```python
from build123d import *

# Parameters (mm, degrees)
SKETCH1_W                   = 60
SKETCH1_H                   = 60
BOSS_EXTRUDE1_DEPTH         = 45
BOSS_EXTRUDE2_DEPTH         = 34
SKETCH3_R                   = 3.5
BOSS_EXTRUDE3_DEPTH         = 4
SKETCH4_R                   = 4.5
BOSS_EXTRUDE4_DEPTH         = 1.5
SKETCH5_R                   = 0.5
BOSS_EXTRUDE5_DEPTH         = 8.5
SKETCH6_R                   = 27
CUT_EXTRUDE1_DEPTH          = 0.3
SKETCH7_R                   = 12
BOSS_EXTRUDE6_DEPTH         = 3.3
SKETCH8_R                   = 4
BOSS_EXTRUDE7_DEPTH         = 29
CUT_EXTRUDE2_DEPTH          = 109.592080743
CUT_EXTRUDE2_DEPTH_BACK     = 109.592080743
M4_TAPPED_HOLE1_D           = 3.3
M4_TAPPED_HOLE1_DEPTH       = 10.1
M4_TAPPED_HOLE1_CSINK_D     = 4
M4_TAPPED_HOLE1_CSINK_ANGLE = 90
M4_TAPPED_HOLE1_TIP         = 0.991420021
FILLET1_R                   = 3.5
FILLET2_R                   = 4
FILLET3_R                   = 5.7


with BuildPart() as part:
    # Sketch1 → Boss-Extrude1 (new body)
    with BuildSketch(Plane(origin=(0, 0, 0), x_dir=(0, 0, -1), z_dir=(1, 0, 0))):
        with Locations((30, 0)):
            Rectangle(SKETCH1_W, SKETCH1_H)
    extrude(amount=-BOSS_EXTRUDE1_DEPTH)

    # Sketch2 → Boss-Extrude2 (add)
    with BuildSketch(Plane.ZY.offset(45)):
        Polygon((-1.8, 16.87), (-1.8, -16.87), (-10.698224855, -19.301775145), (-13.13, -28.2), (-46.87, -28.2), (-49.301775145, -19.301775145), (-58.2, -16.87), (-58.2, 16.87), (-49.301775145, 19.301775145), (-46.87, 28.2), (-13.13, 28.2), (-10.698224855, 19.301775145), align=None)
    extrude(amount=BOSS_EXTRUDE2_DEPTH)

    # Sketch3 → Boss-Extrude3 (add)
    with BuildSketch(Plane.ZY.offset(45)):
        with Locations((-5.251262658, 24.748737342)):
            Circle(SKETCH3_R)
        with Locations((-5.251262658, -24.748737342)):
            Circle(SKETCH3_R)
        with Locations((-54.748737342, -24.748737342)):
            Circle(SKETCH3_R)
        with Locations((-54.748737342, 24.748737342)):
            Circle(SKETCH3_R)
    extrude(amount=BOSS_EXTRUDE3_DEPTH)

    # Sketch4 → Boss-Extrude4 (add)
    with BuildSketch(Plane(origin=(0, 0, -58.2), x_dir=(-1, 0, 0), z_dir=(0, 0, -1))):
        with Locations(Location((71, 0, 0), (0, 0, 180))):
            Circle(SKETCH4_R)
    extrude(amount=BOSS_EXTRUDE4_DEPTH)

    # Sketch5 → Boss-Extrude5 (add)
    with BuildSketch(Plane(origin=(0, 0, -59.7), x_dir=(-1, 0, 0), z_dir=(0, 0, -1))):
        with Locations((73, -2)):
            Circle(SKETCH5_R)
        with Locations((73, 0)):
            Circle(SKETCH5_R)
        with Locations((73, 2)):
            Circle(SKETCH5_R)
        with Locations((69, -2)):
            Circle(SKETCH5_R)
        with Locations((69, 0)):
            Circle(SKETCH5_R)
        with Locations((69, 2)):
            Circle(SKETCH5_R)
    extrude(amount=BOSS_EXTRUDE5_DEPTH)

    # Sketch6 → Cut-Extrude1 (cut)
    with BuildSketch(Plane(origin=(0, 0, 0), x_dir=(0, 0, -1), z_dir=(1, 0, 0))):
        with Locations((30, 0)):
            Circle(SKETCH6_R)
    extrude(amount=-CUT_EXTRUDE1_DEPTH, mode=Mode.SUBTRACT)

    # Sketch7 → Boss-Extrude6 (add)
    with BuildSketch(Plane(origin=(-0.3, 0, 0), x_dir=(0, 0, -1), z_dir=(1, 0, 0))):
        with Locations((20, 0)):
            Circle(SKETCH7_R)
    extrude(amount=BOSS_EXTRUDE6_DEPTH)

    # Sketch8 → Boss-Extrude7 (add)
    with BuildSketch(Plane(origin=(3, 0, 0), x_dir=(0, 0, -1), z_dir=(1, 0, 0))):
        with Locations(Location((20, 0, 0), (0, 0, 180))):
            Circle(SKETCH8_R)
    extrude(amount=BOSS_EXTRUDE7_DEPTH)

    # Sketch9 → Cut-Extrude2 (cut, two sides: drawn at the far end of the back side and taken through both)
    with BuildSketch(Plane(origin=(0, 0, 0), x_dir=(1, 0, 0), z_dir=(0, 1, 0)).offset(-CUT_EXTRUDE2_DEPTH_BACK)):
        with BuildLine():
            Line((32, 17), (20, 17))
            ThreePointArc((20, 17), (17.4, 16.747644855), (14.897059671, 16))
            Line((14.897059671, 16), (32, 16))
            Line((32, 16), (32, 17))
        make_face()
    extrude(amount=CUT_EXTRUDE2_DEPTH + CUT_EXTRUDE2_DEPTH_BACK, mode=Mode.SUBTRACT)

    # M4 Tapped Hole1
    with Locations(Plane(origin=(0, 0, 0), x_dir=(0, 0, -1), z_dir=(1, 0, 0))):
        with Locations((5.251262658, -24.748737342), (5.251262658, 24.748737342), (54.748737342, -24.748737342), (54.748737342, 24.748737342)):
            CounterSinkHole(M4_TAPPED_HOLE1_D / 2, M4_TAPPED_HOLE1_CSINK_D / 2, depth=M4_TAPPED_HOLE1_DEPTH, counter_sink_angle=M4_TAPPED_HOLE1_CSINK_ANGLE)
            with Locations((0, 0, -(M4_TAPPED_HOLE1_DEPTH + M4_TAPPED_HOLE1_TIP / 2))):  # 118° drill point
                Cone(0, M4_TAPPED_HOLE1_D / 2, M4_TAPPED_HOLE1_TIP, mode=Mode.SUBTRACT)

    # Fillet1
    fillet1_edges = [part.edges().sort_by_distance(p)[0] for p in [
        (-62, 16.87, -1.8),
        (-62, 28.2, -13.13),
        (-62, 28.2, -46.87),
        (-62, 16.87, -58.2),
        (-62, -16.87, -58.2),
        (-62, -28.2, -46.87),
        (-62, -28.2, -13.13),
        (-62, -16.87, -1.8),
    ]]
    fillet(fillet1_edges, radius=FILLET1_R)

    # Fillet2
    fillet2_edges = [part.edges().sort_by_distance(p)[0] for p in [
        (-62, 19.301775145, -10.698224855),
        (-62, 19.301775145, -49.301775145),
        (-62, -19.301775145, -49.301775145),
        (-62, -19.301775145, -10.698224855),
    ]]
    fillet(fillet2_edges, radius=FILLET2_R)

    # Fillet3
    fillet3_edges = [part.edges().sort_by_distance(p)[0] for p in [
        (-22.5, 30, 0),
        (-22.5, 30, -60),
        (-22.5, -30, -60),
        (-22.5, -30, 0),
    ]]
    fillet(fillet3_edges, radius=FILLET3_R)


solid = part.part
```
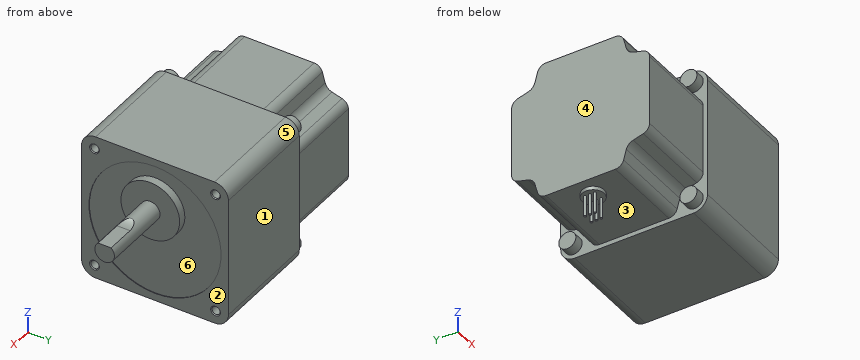
Here's how the part is built. I have some questions about the finished solid (model axes, mm). Face numbers are marked on the shaded views. A direction names the side the tool comes from. Round coordinates to 2 decimals unless told otherwise and drop trailing zeros. Order: outer loops, then holes, each group sorted by start corner. A loop starts at its lowest first (then second) coordinate and runs counter-clockwise, first axis right, second up. Notation, with made-up numbers: (8.5, 77.5) -> (36.5, 77.5) arc R16 ccw to (36.5, 86.5) -> close; hole circle Ø6 at (-38, 11.5). An arc over 180 degrees is marked (long way). Use a Markdown table: item, result. Add a question column.
(1) Suppose I cut it at B-B, the plane y = -9. Please give me the cut outline in (x, z), and give its area (3 significant figures).
(2) For the marked faces 5 and 6, which set-ups out of +Z, -Z, +X, -X, +Y, -Y let a thin tool reach every point of the face, with its end or its side?
(3) Suppose I cut it at C-C, the plane z = -21.5. Please give me the cut outline in (x, y), and give its area (3 significant figures).
(4) If we mould it in two halves opening along X, with no side actions, what happens to the marked faces 1, 2, 3 and 4? For each: released by +X, released by -X, zero draft, split by the parting line, or undercut.
(5) Suppose I cut it at D-D, the plane x = -52. Please give me the cut outline in (y, z), and give its area (3 significant figures).
(6) Suppose I cut it at A-A, the plane x = -25. Please give me the cut outline in (y, z), and give its area (3 significant figures).
(7) I need wall thicknesses on line 1 along Y through (x, z) = (-0.05, -30); line 2 along Z through (x, y) = (-40, -10); line 3 along Z through (x, y) = (-60, -8.5). Which ranges of each line are inside material? Lowest first, please.
(8) For pin 1 Ø3 at (y, z) = (24.75, -54.75) entering from +X; pin 2 Ø2.5 at (y, z) = (24.75, -5.25) entering from -X; pin 3 Ø8 at (x, y) = (-20.5, -21) entering from -Z, each with a flat end and sliding along its axis, tell me the tip position at first contact or that it passes through.
Verdict:
| question | item | result |
|---|---|---|
| 1 | outline | (-79, -58.2) -> (-45, -58.2) -> (-45, -60) -> (0, -60) -> (0, -55.46) -> (-0.3, -55.46) -> (-0.3, -27.94) -> (3, -27.94) -> (3, -12.06) -> (-0.3, -12.06) -> (-0.3, -4.54) -> (0, -4.54) -> (0, 0) -> (-45, 0) -> (-45, -1.8) -> (-79, -1.8) -> close |
| 1 | area | 4,650 mm2 |
| 2 | face 5 | +Z, +X, -X, +Y |
| 2 | face 6 | +X |
| 3 | outline | (-79, -28.2) -> (-45, -28.2) -> (-45, -30) -> (0, -30) -> (0, -25.63) -> (-0.3, -25.63) -> (-0.3, -11.91) -> (3, -11.91) -> (3, -3.71) -> (32, -3.71) -> (32, 3.71) -> (3, 3.71) -> (3, 11.91) -> (-0.3, 11.91) -> (-0.3, 25.63) -> (0, 25.63) -> (0, 30) -> (-45, 30) -> (-45, 28.2) -> (-79, 28.2) -> close |
| 3 | area | 4,900 mm2 |
| 4 | face 1 | zero draft |
| 4 | face 2 | released by +X |
| 4 | face 3 | undercut |
| 4 | face 4 | released by -X |
| 5 | outline | (-28.2, -44.2) arc R3.5 ccw to (-25.62, -47.57) -> (-21.5, -48.7) arc R4 cw to (-18.7, -51.5) -> (-17.57, -55.62) arc R3.5 ccw to (-14.2, -58.2) -> (14.2, -58.2) arc R3.5 ccw to (17.57, -55.62) -> (18.7, -51.5) arc R4 cw to (21.5, -48.7) -> (25.62, -47.57) arc R3.5 ccw to (28.2, -44.2) -> (28.2, -15.8) arc R3.5 ccw to (25.62, -12.43) -> (21.5, -11.3) arc R4 cw to (18.7, -8.5) -> (17.57, -4.38) arc R3.5 ccw to (14.2, -1.8) -> (-14.2, -1.8) arc R3.5 ccw to (-17.57, -4.38) -> (-18.7, -8.5) arc R4 cw to (-21.5, -11.3) -> (-25.62, -12.43) arc R3.5 ccw to (-28.2, -15.8) -> close |
| 5 | area | 2,770 mm2 |
| 6 | outline | (-30, -54.3) arc R5.7 ccw to (-24.3, -60) -> (24.3, -60) arc R5.7 ccw to (30, -54.3) -> (30, -5.7) arc R5.7 ccw to (24.3, 0) -> (-24.3, 0) arc R5.7 ccw to (-30, -5.7) -> close |
| 6 | area | 3,570 mm2 |
| 7 | line 1 | -30 to -27, -6.63 to 6.63, 27 to 30 |
| 7 | line 2 | -60 to 0 |
| 7 | line 3 | -58.2 to -1.8 |
| 8 | pin 1 | x = -10.19 |
| 8 | pin 2 | x = -49 |
| 8 | pin 3 | z = -60 |
